For this review, take the finished solid that the model builds, in its own axes (mm). Face numbers are marked on the shaded views. A direction names the side the tool comes from. Coordinates: 2 decimals unless noted, no trailing zeros. Loops run counter-clockwise (first coordinate to the right, second up) from the corner with the lowest first, then second, coordinate; pieces in that order, holes last. Notation, with made-up numbers: (-22.75, 53) - (7.25, 53) arc R35 ccw to (7.25, 90) - close; hole circle Ø4 at (3, -26). An arc over 180 degrees is marked (long way). Use one line per item in the form item = value. Start each with the question number.
1. Draft analysis for pull direction X (two halves, no side actions). For the marked faces 1, 2 and 3, state which applies: +X half, -X half, draft (parallel to the pull), parting line (faces both ways), or undercut.
2. Add section C-C on z = 46.5. Give the boundary of the cut face in (x, y), and give its area (3 significant figures).
3. Add section A-A on x = -1.5. Give the boundary of the cut face in (y, z).
4. Machinability: for the marked faces 4, 5 and 6, which of the approach directions +Z, -Z, +X, -X, +Y, -Y give a long, thin tool a straight path to every point of the face, cutting with its end or side? Answer none if there is none.
5. To check wall thickness, follow probe 1 along X at (y, z) = (30, 9); probe 2 along X at (y, z) = (8, -21.5); probe 3 along Z at (x, y) = (-36.5, 25). State the ranges of each line that lie inside material, in increasing order.
6. For pin 1 Ø15.5 at (y, z) = (21, 12) entering from +X; pin 2 Ø6 at (x, y) = (-20, 16.5) entering from +Z; pin 3 Ø15.5 at (x, y) = (-9.5, 23) entering from -Z, all flat-tipped, find the tip position at first contact; note any pin that passes through.
7. Add section B-B on y = 43. Give the boundary of the cut face in (x, z).
8. Add section D-D on y = 34.5. Give the boundary of the cut face in (x, z).
```python
from build123d import *

# Parameters (mm, degrees)
SKETCH1_W           = 60
SKETCH1_H           = 60
BOSS_EXTRUDE1_DEPTH = 51.95
SKETCH3_W           = 5
SKETCH3_H           = 40
BOSS_EXTRUDE2_DEPTH = 18
SKETCH4_W           = 5
SKETCH4_H           = 40
BOSS_EXTRUDE3_DEPTH = 30
SKETCH5_W           = 5
SKETCH5_H           = 40
BOSS_EXTRUDE4_DEPTH = 50
SKETCH6_W           = 5
SKETCH6_H           = 40
BOSS_EXTRUDE5_DEPTH = 30
SKETCH7_W           = 25
SKETCH7_H           = 25
CUT_EXTRUDE1_DEPTH  = 52.95
FILLET1_R           = 3
FILLET2_R           = 5
FILLET3_R           = 5


with BuildPart() as part:
    # Sketch1 → Boss-Extrude1 (new body)
    with BuildSketch(Plane(origin=(0, 0, 0), x_dir=(1, 0, 0), z_dir=(0, 1, 0))):
        Rectangle(SKETCH1_W, SKETCH1_H)
    extrude(amount=BOSS_EXTRUDE1_DEPTH)

    # Sketch3 → Boss-Extrude2 (add)
    with BuildSketch(Plane(origin=(0, 0, -30), x_dir=(-1, 0, 0), z_dir=(0, 0, -1))):
        with Locations((-27.5, 20)):
            Rectangle(SKETCH3_W, SKETCH3_H)
    extrude(amount=BOSS_EXTRUDE2_DEPTH)

    # Sketch4 → Boss-Extrude3 (add)
    with BuildSketch(Plane(origin=(30, 0, 0), x_dir=(0, 0, -1), z_dir=(1, 0, 0))):
        with Locations((45.5, 20)):
            Rectangle(SKETCH4_W, SKETCH4_H)
    extrude(amount=BOSS_EXTRUDE3_DEPTH)

    # Sketch5 → Boss-Extrude4 (add)
    with BuildSketch(Plane.ZY.offset(30)):
        with Locations((27.5, 20)):
            Rectangle(SKETCH5_W, SKETCH5_H)
    extrude(amount=BOSS_EXTRUDE4_DEPTH)

    # Sketch6 → Boss-Extrude5 (add)
    with BuildSketch(Plane.XY.offset(30)):
        with Locations((-77.5, 20)):
            Rectangle(SKETCH6_W, SKETCH6_H)
    extrude(amount=BOSS_EXTRUDE5_DEPTH)

    # Sketch7 → Cut-Extrude1 (cut, through all)
    with BuildSketch(Plane(origin=(0, 51.95, 0), x_dir=(1, 0, 0), z_dir=(0, 1, 0))):
        Rectangle(SKETCH7_W, SKETCH7_H)
    extrude(amount=-CUT_EXTRUDE1_DEPTH, mode=Mode.SUBTRACT)

    # Fillet1
    fillet1_edges = [part.edges().sort_by_distance(p)[0] for p in [
        (12.5, 25.975, -12.5),
        (12.5, 25.975, 12.5),
        (-12.5, 25.975, 12.5),
        (-12.5, 25.975, -12.5),
    ]]
    fillet(fillet1_edges, radius=FILLET1_R)

    # Fillet2
    fillet2_edges = [part.edges().sort_by_distance(p)[0] for p in [
        (30, 20, -43),
        (-75, 20, 30),
    ]]
    fillet(fillet2_edges, radius=FILLET2_R)

    # Fillet3
    fillet3_edges = [part.edges().sort_by_distance(p)[0] for p in [
        (25, 20, -30),
        (-30, 20, 25),
    ]]
    fillet(fillet3_edges, radius=FILLET3_R)


solid = part.part
```
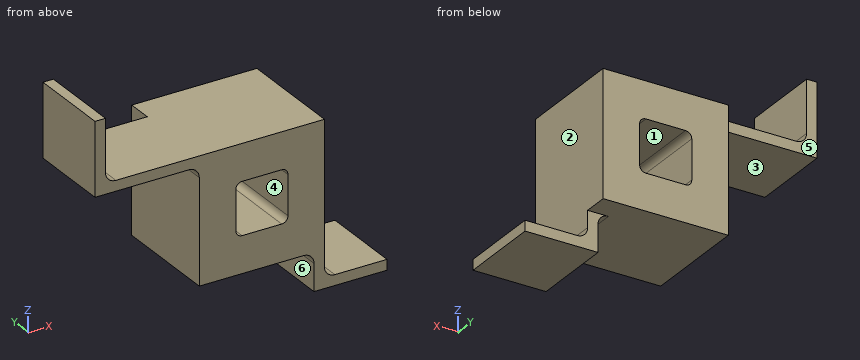
Conclusion:
q1.face_1 = undercut
q1.face_2 = +X half
q1.face_3 = draft
q2.outline = (-80, 0) - (-75, 0) - (-75, 40) - (-80, 40) - close
q2.area = 200 mm^2
q3.outline = (0, -30) - (51.95, -30) - (51.95, -12.5) - (0, -12.5) - close; (0, 12.5) - (51.95, 12.5) - (51.95, 30) - (0, 30) - close
q4.face_4 = +Y, -Y
q4.face_5 = +Z, -Z, -X, +Y
q4.face_6 = -Z, -X, +Y, -Y
q5.probe_1 = -30 to -12.5, 12.5 to 30
q5.probe_2 = -30 to 30
q5.probe_3 = 25 to 30
q6.pin_1 = 30
q6.pin_2 = 30
q6.pin_3 = -30
q7.outline = (-30, -30) - (30, -30) - (30, 30) - (-30, 30) - close; hole (-12.5, -9.5) arc R3 ccw to (-9.5, -12.5) - (9.5, -12.5) arc R3 ccw to (12.5, -9.5) - (12.5, 9.5) arc R3 ccw to (9.5, 12.5) - (-9.5, 12.5) arc R3 ccw to (-12.5, 9.5) - close
q8.outline = (-80, 25) - (-35, 25) arc R5 cw to (-30, 20) - (-30, -30) - (20, -30) arc R5 cw to (25, -35) - (25, -48) - (60, -48) - (60, -43) - (35, -43) arc R5 cw to (30, -38) - (30, 30) - (-70, 30) arc R5 cw to (-75, 35) - (-75, 60) - (-80, 60) - close; hole (-12.5, -9.5) arc R3 ccw to (-9.5, -12.5) - (9.5, -12.5) arc R3 ccw to (12.5, -9.5) - (12.5, 9.5) arc R3 ccw to (9.5, 12.5) - (-9.5, 12.5) arc R3 ccw to (-12.5, 9.5) - close
